Geometry check sheet. Reference: the model listing, model coordinates, mm. Face numbers are marked on the shaded views. A direction names the side the tool comes from. Coordinates: 2 decimals unless noted, no trailing zeros. Write each loop counter-clockwise with the first axis right and the second up, starting at its lowest first coordinate (ties: lowest second). Pieces come first, ordered by that corner, then holes.
from build123d import *

# Parameters (mm, degrees)
F1_R     = 11
F1_R_2   = 8
F2_DEPTH = 7
F3_COUNT = 5


with BuildPart() as f2:
    # F1 (on Top) → F2 (new body)
    with BuildSketch(Plane.XY):
        with BuildLine():
            ThreePointArc((-14, 0), (0, -14), (14, 0))
            ThreePointArc((14, 0), (9.8994949366, 9.8994949366), (0, 14))
            ThreePointArc((0, 14), (-9.8994949366, 9.8994949366), (-14, 0))
        make_face()
        Circle(F1_R, mode=Mode.SUBTRACT)
        with BuildLine():
            ThreePointArc((-14, 0), (-9.8994949366, 9.8994949366), (0, 14))
            ThreePointArc((0, 14), (0.0928065847, 20.9641089066), (4.7098193128, 26.1785714286))
            ThreePointArc((4.7098193128, 26.1785714286), (-6.9834201124, 27.8423576834), (-8.9347861793, 39.4910573288))
            ThreePointArc((-8.9347861793, 39.4910573288), (-14.8385397391, 20.1779196855), (-14, 0))
        make_face()
        with BuildLine():
            ThreePointArc((-8.9347861793, 39.4910573288), (-6.9834201124, 27.8423576834), (4.7098193128, 26.1785714286))
            ThreePointArc((4.7098193128, 26.1785714286), (8.5760769915, 29.8569558201), (10, 35))
            ThreePointArc((10, 35), (2.307827789, 44.730052975), (-8.9347861793, 39.4910573288))
        make_face()
        with Locations((0, 35)):
            Circle(F1_R_2, mode=Mode.SUBTRACT)
    extrude(amount=F2_DEPTH)

    # F3: F2 ×5 about axis
    f3_axis = Axis((0, 0, 7), (0, 0, 1))


with BuildPart() as f2_1:
    add(f2.part)
    for i in range(1, F3_COUNT):
        add(f2.part.rotate(f3_axis, i * 360 / F3_COUNT))


solid = f2_1.part
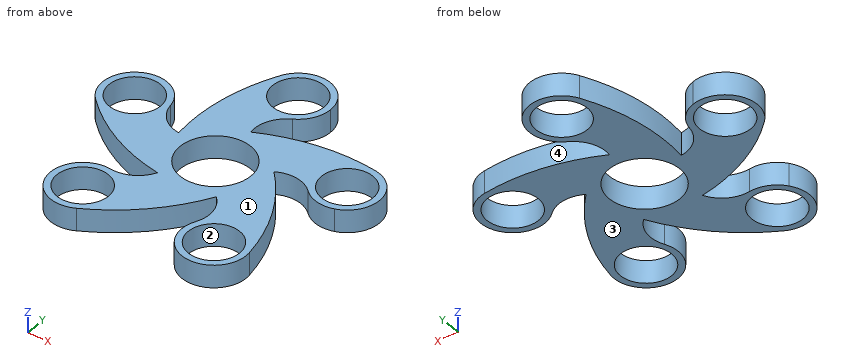
1. Gauge pin test, flat ends, axial feed: pin 1 Ø3 at (x, z) = (-7.5, 2) entering from -Y; pin 2 Ø14.5 at (x, y) = (33.29, 10.82) entering from -Z. Record the tip position at first contact, or that the pin passes through.
Computed values:
pin 1: stops at y = -32.97
pin 2: passes through
2. Sectioned sample at A-A, the plane z = 6. Record the boundary of the cut face in (x, y), and give its area (3 significant figures).
Computed values:
outline: (-40.32, 3.71) arc R60 ccw to (-8.74, -12.69) arc R10 cw to (-19.2, -18.41) arc R10 ccw (long way) to (-15.98, -37.2) arc R60 ccw to (9.37, -12.23) arc R10 cw to (11.58, -23.95) arc R10 ccw (long way) to (30.44, -26.7) arc R60 ccw to (14.53, 5.13) arc R10 cw to (26.35, 3.61) arc R10 ccw (long way) to (34.8, 20.7) arc R60 ccw to (-0.39, 15.4) arc R10 cw to (4.71, 26.18) arc R10 ccw (long way) to (-8.93, 39.49) arc R60 ccw to (-14.77, 4.39) arc R10 cw to (-23.44, 12.57) arc R10 ccw (long way) to start; hole circle Ø16 at (-33.29, 10.82); hole circle Ø16 at (-20.57, -28.32); hole circle Ø22 at (0, 0); hole circle Ø16 at (0, 35); hole circle Ø16 at (20.57, -28.32); hole circle Ø16 at (33.29, 10.82)
area: 2,140 mm2
3. Draft check along Y on the marked faces 1 and 2. Enter one of: released by +Y, released by -Y, zero draft, split by the parting line, or undercut.
Computed values:
face 1: zero draft
face 2: undercut
4. Access from +Z, -Z, +X, -X, +Y, -Y to the whole of each face (thin tool, end or side, straight path). Record for the marked faces 3 and 4.
Computed values:
face 3: -Z, +X, -X, +Y, -Y
face 4: +Z, -Z
5. Sectioned sample at B-B, the plane y = 29. Record the boundary of the cut face in (x, z).
Computed values:
outline: (-13.03, 0) - (-5.29, 0) - (-5.29, 7) - (-13.03, 7) - close; (5.29, 0) - (8, 0) - (8, 7) - (5.29, 7) - close
6. Thickness scan on line 1 along Y through (x, z) = (18, 1.75); line 2 along Y through (x, z) = (-20, 5.5); line 3 along Y through (x, z) = (1, 4). Record the ranges inside material, lowest first.
Computed values:
line 1: y = -37.98 to -35.89, -20.74 to 1.18, 6.3 to 20.89
line 2: y = -38.3 to -36.3, -20.34 to -18.33, -9.51 to 6.64
line 3: y = -24.12 to -10.95, 10.95 to 16.05, 22.75 to 27.06, 42.94 to 44.95
7. Sectioned sample at C-C, the plane x = -3. Record the boundary of the cut face in (y, z).
Computed values:
outline: (-28.15, 0) - (-10.58, 0) - (-10.58, 7) - (-28.15, 7) - close; (10.58, 0) - (27.58, 0) - (27.58, 7) - (10.58, 7) - close; (42.42, 0) - (44.54, 0) - (44.54, 7) - (42.42, 7) - close
